Source: CAD feature listing. Evaluate the final solid. Frame: model axes, mm. Face numbers are marked on the shaded views. A direction names the side the tool comes from. Give positions to 0.01 mm unless a question says otherwise; leave off trailing zeros. Order: outer loops, then holes, each group sorted by start corner. A loop starts at its lowest first (then second) coordinate and runs counter-clockwise, first axis right, second up. Notation, with made-up numbers: M 89,24 L 101,24 A20 ccw 101,55 Z; hole C -12,82 d4. An arc over 180 degrees is marked long. Use CSV: the item, a comma, the result in double quotes. Start each with the question number.
Item 1: First-contact query: pin 1 (10 mm diameter, centred on y = 74, z = 82, fed in from +X); pin 2 (7.5 mm diameter, centred on x = 40, z = 127, fed in from -Y) (3 decimals). Flat tips, straight axial feed; report the tip coordinate or a pass-through.
Item 2: Section query A-A on z = 127. Return loops of the section in (x, y) (3 decimals), and give its area (3 significant figures).
Item 3: Section query C-C on x = 59. Return loops of the section in (y, z), and give its area (3 significant figures).
Item 4: Ray query, probe 1 along Y at (x, z) = (15, 128.5); probe 2 along Z at (x, y) = (40, 3.9); probe 3 along X at (y, z) = (4.45, 127). Return the intervals inside material, ascending. Write a range as from..to.
Item 5: Access query for the marked faces 1 and 2. Directions: +Z, -Z, +X, -X, +Y, -Y. A direction counts if a zero-diameter tool reaches every point of the face in a straight line with its end or side. Return the directions, or none.
Item 6: Section query B-B on x = 40. Return loops of the section in (y, z) (3 decimals).
Item 7: Section query D-D on z = 35.5. Return loops of the section in (x, y), and give its area (3 significant figures).
from build123d import *

# Parameters (mm, degrees)
EXTRUDE_1_DEPTH             = 202
HOLE_WIZARD_M61_D           = 6.6
HOLE_WIZARD_M61_DEPTH       = 10
HOLE_WIZARD_M61_CSINK_D     = 13.71
HOLE_WIZARD_M61_CSINK_ANGLE = 90
HOLE_WIZARD_M61_TIP         = 1.982840043


with BuildPart() as part:
    # Эскиз1 → Бобышка-Вытянуть1 (new body)
    with BuildSketch(Plane.XY):
        with BuildLine():
            Line((70, 0), (8, 0))
            ThreePointArc((8, 0), (2.343145751, 2.343145751), (0, 8))
            Line((0, 8), (0, 302))
            ThreePointArc((0, 302), (2.343145751, 307.656854249), (8, 310))
            Line((8, 310), (70, 310))
            Line((70, 310), (70, 305))
            Line((70, 305), (8, 305))
            ThreePointArc((8, 305), (5.878679656, 304.121320344), (5, 302))
            Line((5, 302), (5, 8))
            ThreePointArc((5, 8), (5.878679656, 5.878679656), (8, 5))
            Line((8, 5), (70, 5))
            Line((70, 5), (70, 0))
        make_face()
    extrude(amount=EXTRUDE_1_DEPTH)

    # Зенковка для винта с потайной головкой и внутренним шестигранником M61
    with Locations(Plane.XZ):
        with Locations((40, 127)):
            CounterSinkHole(HOLE_WIZARD_M61_D / 2, HOLE_WIZARD_M61_CSINK_D / 2, depth=HOLE_WIZARD_M61_DEPTH, counter_sink_angle=HOLE_WIZARD_M61_CSINK_ANGLE)
            with Locations((0, 0, -(HOLE_WIZARD_M61_DEPTH + HOLE_WIZARD_M61_TIP / 2))):  # 118° drill point
                Cone(0, HOLE_WIZARD_M61_D / 2, HOLE_WIZARD_M61_TIP, mode=Mode.SUBTRACT)


solid = part.part
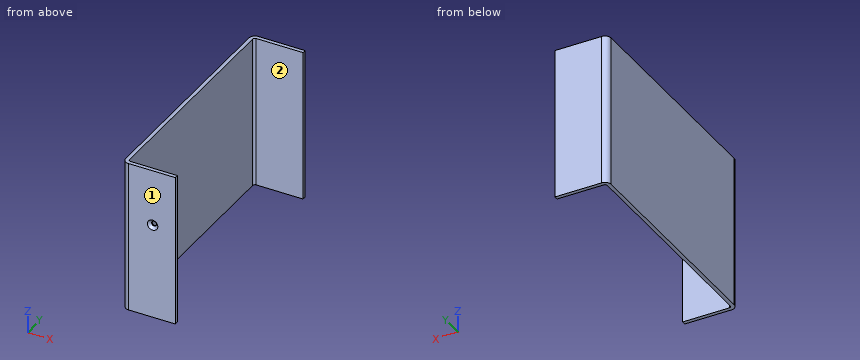
Verdict:
1,pin 1,"x = 5"
1,pin 2,"y = 3.105"
2,outline,"M 0,8 A8 ccw 8,0 L 33.145,0 L 36.7,3.555 L 36.7,5 L 8,5 A3 cw 5,8 L 5,302 A3 cw 8,305 L 70,305 L 70,310 L 8,310 A8 ccw 0,302 Z; M 43.3,3.555 L 46.855,0 L 70,0 L 70,5 L 43.3,5 Z"
2,area,"2,130 mm2"
3,outline,"M 0,0 L 5,0 L 5,202 L 0,202 Z; M 305,0 L 310,0 L 310,202 L 305,202 Z"
3,area,"2,020 mm2"
4,probe 1,"0..5, 305..310"
4,probe 2,"0..123.7, 130.3..202"
4,probe 3,"0.83..36.7, 43.3..70"
5,face 1,"+Z, -Z, +X, -X, -Y"
5,face 2,"+Z, -Z, +X"
6,outline,"M 0,0 L 5,0 L 5,123.7 L 3.555,123.7 L 0,120.145 Z; M 0,133.855 L 3.555,130.3 L 5,130.3 L 5,202 L 0,202 Z; M 305,0 L 310,0 L 310,202 L 305,202 Z"
7,outline,"M 0,8 A8 ccw 8,0 L 70,0 L 70,5 L 8,5 A3 cw 5,8 L 5,302 A3 cw 8,305 L 70,305 L 70,310 L 8,310 A8 ccw 0,302 Z"
7,area,"2,180 mm2"
